```python
from build123d import *

# Parameters (mm, degrees)
ESQUISSE1_R        = 12.6
BOSS_EXTRU_1_DEPTH = 6


with BuildPart() as part:
    # Esquisse1 → Boss.-Extru.1 (new body)
    with BuildSketch(Plane.XY):
        with BuildLine():
            ThreePointArc((-85.542599785, 135.212660731), (-106.965290191, 118.9891873), (-125.370670455, 99.409229902))
            ThreePointArc((-125.370670455, 99.409229902), (-124.062234057, 84.312289025), (-138.580667025, 79.971236872))
            ThreePointArc((-138.580667025, 79.971236872), (-150.010093296, 55.650443927), (-157.207988245, 29.759845967))
            ThreePointArc((-157.207988245, 29.759845967), (-149.0335271, 17.000229412), (-159.871573528, 6.409366404))
            ThreePointArc((-159.871573528, 6.409366404), (-158.689391845, -20.43714549), (-153.03085049, -46.707160034))
            ThreePointArc((-153.03085049, -46.707160034), (-139.863035133, -54.206377884), (-144.537829197, -68.620812667))
            ThreePointArc((-144.537829197, -68.620812667), (-131.014863137, -91.84283117), (-113.796189109, -112.474118553))
            ThreePointArc((-113.796189109, -112.474118553), (-98.651607349, -112.994957265), (-96.092210067, -127.930790526))
            ThreePointArc((-96.092210067, -127.930790526), (-73.326408184, -142.208431054), (-48.492192196, -152.474611972))
            ThreePointArc((-48.492192196, -152.474611972), (-34.840285202, -145.897753674), (-25.633023647, -157.933366008))
            ThreePointArc((-25.633023647, -157.933366008), (1.160243205, -159.995793181), (27.920781555, -157.545009306))
            ThreePointArc((27.920781555, -157.545009306), (36.952526413, -145.377132974), (50.698379579, -151.755310642))
            ThreePointArc((50.698379579, -151.755310642), (75.381096858, -141.130047249), (97.937440733, -126.523743632))
            ThreePointArc((97.937440733, -126.523743632), (100.279959554, -111.552363094), (115.415395025, -110.811942457))
            ThreePointArc((115.415395025, -110.811942457), (132.333049661, -89.933108294), (145.517812514, -66.517413067))
            ThreePointArc((145.517812514, -66.517413067), (140.634462465, -52.172291181), (153.692134377, -44.482893684))
            ThreePointArc((153.692134377, -44.482893684), (158.969095574, -18.13357804), (159.761807127, 8.727255209))
            ThreePointArc((159.761807127, 8.727255209), (148.771304855, 19.159823897), (156.759857935, 32.036649955))
            ThreePointArc((156.759857935, 32.036649955), (149.187237475, 57.82013641), (137.406297066, 81.972614492))
            ThreePointArc((137.406297066, 81.972614492), (122.826434191, 86.102654221), (123.9157872, 101.216983173))
            ThreePointArc((123.9157872, 101.216983173), (105.228381173, 120.527954416), (83.572660273, 136.439035672))
            ThreePointArc((83.572660273, 136.439035672), (68.743507673, 133.320404113), (62.684102965, 147.209725343))
            ThreePointArc((62.684102965, 147.209725343), (37.162970883, 155.624270585), (10.59353417, 159.648918048))
            ThreePointArc((10.59353417, 159.648918048), (-1.087728004, 149.996056107), (-12.907753834, 159.478493506))
            ThreePointArc((-12.907753834, 159.478493506), (-39.416028174, 155.068941839), (-64.812442944, 146.285157277))
            ThreePointArc((-64.812442944, 146.285157277), (-70.669778304, 132.309419296), (-85.542599785, 135.212660731))
        make_face()
        Circle(ESQUISSE1_R, mode=Mode.SUBTRACT)
    extrude(amount=BOSS_EXTRU_1_DEPTH)


solid = part.part
```
Verification items for the finished model (mm, model axes). Round coordinates to 2 decimals unless told otherwise and drop trailing zeros. Order: outer loops, then holes, each group sorted by start corner. A loop starts at its lowest first (then second) coordinate and runs counter-clockwise, first axis right, second up. Notation, with made-up numbers: (-9.5, 0.5) -> (12.5, 0.5) arc R25 cw to (12.5, 39.5) -> close; hole circle Ø9 at (30, -39). An arc over 180 degrees is marked (long way). Put each result on its own line as item: value. Start each with the question number.
(1) Section check B-B (z = 5.1). Enter the section's corners in (x, y) (1 decimal).
(2) Draft check along X on faces 1 (the face through (122.96, 85.916, 2.958)), 2 (the face through (-70.5, 132.4, 3)), 3 (the face through (-106.685, 119.241, 2.958)), 4 (the face through (37.529, 155.536, 2.958)). Enter one of: +X half, -X half, draft (parallel to the pull), parting line (faces both ways), or undercut.
(3) Section check D-D (y = -74). Enter the section's corners in (x, z), then the cut area to 3 significant figures.
(4) Section check C-C (x = 0). Enter the section's corners in (y, z), then the cut area to 3 significant figures.
(5) Depth check by flat-ended pin: pin 1 Ø3 at (y, z) = (-77, 2.5) entering from -X; pin 2 Ø2 at (x, z) = (37.5, 4.5) entering from -Y; pin 3 Ø4 at (x, y) = (4.5, 18) entering from -Z. Enter the tip coordinate at first touch or a pass-through.
(6) Section check A-A (y = 0). Enter the section's corners in (x, z), then the cut area to 3 significant figures.
(7) Material ranges on line 1 along Y through (x, z) = (0, 3.1); line 2 along X through (y, z) = (92.5, 4.7); line 3 along X through (y, z) = (4.5, 4.6), recorded low to high.
Completed:
1. outline: (-159.9, 6.4) arc R160 ccw to (-153, -46.7) arc R12 cw to (-144.5, -68.6) arc R160 ccw to (-113.8, -112.5) arc R12 cw to (-96.1, -127.9) arc R160 ccw to (-48.5, -152.5) arc R12 cw to (-25.6, -157.9) arc R160 ccw to (27.9, -157.5) arc R12 cw to (50.7, -151.8) arc R160 ccw to (97.9, -126.5) arc R12 cw to (115.4, -110.8) arc R160 ccw to (145.5, -66.5) arc R12 cw to (153.7, -44.5) arc R160 ccw to (159.8, 8.7) arc R12 cw to (156.8, 32) arc R160 ccw to (137.4, 82) arc R12 cw to (123.9, 101.2) arc R160 ccw to (83.6, 136.4) arc R12 cw to (62.7, 147.2) arc R160 ccw to (10.6, 159.6) arc R12 cw to (-12.9, 159.5) arc R160 ccw to (-64.8, 146.3) arc R12 cw to (-85.5, 135.2) arc R160 ccw to (-125.4, 99.4) arc R12 cw to (-138.6, 80) arc R160 ccw to (-157.2, 29.8) arc R12 cw to start; hole circle Ø25.2 at (0, 0)
2. face 1: undercut
2. face 2: undercut
2. face 3: -X half
2. face 4: +X half
3. outline: (-141.86, 0) -> (141.86, 0) -> (141.86, 6) -> (-141.86, 6) -> close
3. area: 1,700 mm2
4. outline: (-160, 0) -> (-12.6, 0) -> (-12.6, 6) -> (-160, 6) -> close; (12.6, 0) -> (150.05, 0) -> (150.05, 6) -> (12.6, 6) -> close
4. area: 1,710 mm2
5. pin 1: stops at x = -141.07
5. pin 2: stops at y = -145.5
5. pin 3: stops at z = 0
6. outline: (-160, 0) -> (-12.6, 0) -> (-12.6, 6) -> (-160, 6) -> close; (12.6, 0) -> (160, 0) -> (160, 6) -> (12.6, 6) -> close
6. area: 1,770 mm2
7. line 1: y = -160 to -12.6, 12.6 to 150.05
7. line 2: x = -122.07 to 120.66
7. line 3: x = -159.94 to -11.77, 11.77 to 159.94
